Build history of the part. All positions in model axes, mm. Coordinates: 2 decimals unless noted, no trailing zeros. Order: outer loops, then holes, each group sorted by start corner. A loop starts at its lowest first (then second) coordinate and runs counter-clockwise, first axis right, second up. Notation, with made-up numbers: (51.5, 52) - (102.5, 52) arc R30 ccw to (102.5, 91) - close; hole circle Ø10 at (-33, -36). An arc over 180 degrees is marked (long way). Return JSON: item names as keys, results as strings.
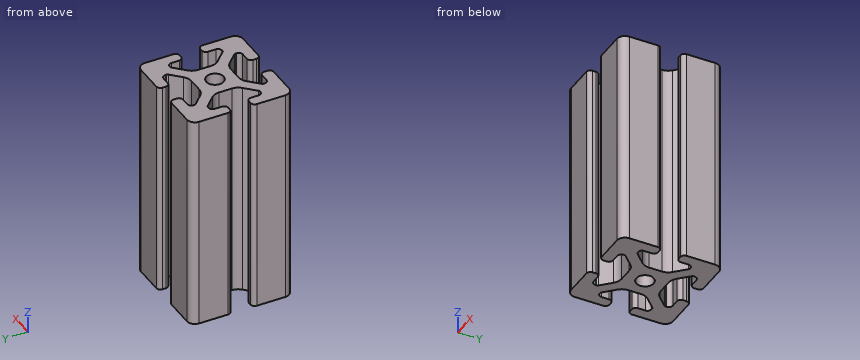
from build123d import *

# Parameters (mm, degrees)
SKETCH1_R      = 3.4
EXTRUDE1_DEPTH = 85.4


with BuildPart() as part:
    # Sketch1 → Extrude1 (new body)
    with BuildSketch(Plane.XY):
        with BuildLine():
            Line((-8.715, -15.524615034), (-5.63, -15.524615034))
            ThreePointArc((-5.63, -15.524615034), (-4.519842354, -15.984457388), (-4.06, -17.094615034))
            Line((-4.06, -17.094615034), (-4.06, -18.43))
            ThreePointArc((-4.06, -18.43), (-4.519842354, -19.540157646), (-5.63, -20))
            Line((-5.63, -20), (-16.674615034, -20))
            ThreePointArc((-16.674615034, -20), (-18.951578385, -19.194274381), (-20, -17.018368134))
            Line((-20, -17.018368134), (-20, -5.757918808))
            ThreePointArc((-20, -5.757918808), (-19.564709668, -4.603883664), (-18.43, -4.120449326))
            Line((-18.43, -4.120449326), (-17.25, -4.120449326))
            ThreePointArc((-17.25, -4.120449326), (-16.115287682, -4.60388249), (-15.67999625, -5.757919334))
            Line((-15.67999625, -5.757919334), (-15.67999625, -8.715399492))
            ThreePointArc((-15.67999625, -8.715399492), (-15.220153896, -9.825557139), (-14.10999625, -10.285399492))
            Line((-14.10999625, -10.285399492), (-13.816898819, -10.285399492))
            ThreePointArc((-13.816898819, -10.285399492), (-13.526061711, -10.227547119), (-13.279501941, -10.062800646))
            Line((-13.279501941, -10.062800646), (-9.076242789, -5.859541495))
            ThreePointArc((-9.076242789, -5.859541495), (-8.046572221, -4.318530588), (-7.685, -2.500784284))
            Line((-7.685, -2.500784284), (-7.685, 2.500784284))
            ThreePointArc((-7.685, 2.500784284), (-8.046572221, 4.318530588), (-9.076242789, 5.859541495))
            Line((-9.076242789, 5.859541495), (-13.040489136, 9.823787841))
            ThreePointArc((-13.040489136, 9.823787841), (-13.354224618, 10.012729352), (-13.71989919, 10.033001362))
            Line((-13.71989919, 10.033001362), (-14.05520779, 10.044710596))
            ThreePointArc((-14.05520779, 10.044710596), (-15.200613642, 9.605030484), (-15.68, 8.475666998))
            Line((-15.68, 8.475666998), (-15.68, 5.572979049))
            ThreePointArc((-15.68, 5.572979049), (-16.139842354, 4.462821403), (-17.25, 4.002979049))
            Line((-17.25, 4.002979049), (-18.43, 4.002979049))
            ThreePointArc((-18.43, 4.002979049), (-19.540157646, 4.462821403), (-20, 5.572979049))
            Line((-20, 5.572979049), (-20, 13.004526564))
            Line((-20, 13.004526564), (-20, 16.83))
            ThreePointArc((-20, 16.83), (-19.071528496, 19.071528496), (-16.83, 20))
            Line((-16.83, 20), (-5.63, 20))
            ThreePointArc((-5.63, 20), (-4.519842354, 19.540157646), (-4.06, 18.43))
            Line((-4.06, 18.43), (-4.06, 17.094615034))
            ThreePointArc((-4.06, 17.094615034), (-4.519842354, 15.984457388), (-5.63, 15.524615034))
            Line((-5.63, 15.524615034), (-8.715, 15.524615034))
            ThreePointArc((-8.715, 15.524615034), (-9.825157646, 15.06477268), (-10.285, 13.954615034))
            Line((-10.285, 13.954615034), (-10.285, 13.492503602))
            ThreePointArc((-10.285, 13.492503602), (-10.227148445, 13.201664194), (-10.062401154, 12.955102448))
            Line((-10.062401154, 12.955102448), (-6.217092793, 9.109794088))
            ThreePointArc((-6.217092793, 9.109794088), (-4.63891877, 8.055291919), (-2.777335583, 7.685))
            Line((-2.777335583, 7.685), (2.777335583, 7.685))
            ThreePointArc((2.777335583, 7.685), (4.63891877, 8.055291919), (6.217092793, 9.109794088))
            Line((6.217092793, 9.109794088), (10.062401154, 12.955102448))
            ThreePointArc((10.062401154, 12.955102448), (10.227148445, 13.201664194), (10.285, 13.492503602))
            Line((10.285, 13.492503602), (10.285, 13.954615034))
            ThreePointArc((10.285, 13.954615034), (9.825157646, 15.06477268), (8.715, 15.524615034))
            Line((8.715, 15.524615034), (5.63, 15.524615034))
            ThreePointArc((5.63, 15.524615034), (4.519842354, 15.984457388), (4.06, 17.094615034))
            Line((4.06, 17.094615034), (4.06, 18.43))
            ThreePointArc((4.06, 18.43), (4.519842354, 19.540157646), (5.63, 20))
            Line((5.63, 20), (12.979635074, 20))
            Line((12.979635074, 20), (16.83, 20))
            ThreePointArc((16.83, 20), (19.071528496, 19.071528496), (20, 16.83))
            Line((20, 16.83), (20, 13.001098436))
            Line((20, 13.001098436), (20, 5.63))
            ThreePointArc((20, 5.63), (19.540157461, 4.519842693), (18.43, 4.060000526))
            Line((18.43, 4.060000526), (17.24999625, 4.060000526))
            ThreePointArc((17.24999625, 4.060000526), (16.139838603, 4.519842879), (15.67999625, 5.630000526))
            Line((15.67999625, 5.630000526), (15.67999625, 8.715399492))
            ThreePointArc((15.67999625, 8.715399492), (15.220153896, 9.825557139), (14.10999625, 10.285399492))
            Line((14.10999625, 10.285399492), (13.816903094, 10.285399492))
            ThreePointArc((13.816903094, 10.285399492), (13.526063686, 10.227547937), (13.279501941, 10.062800646))
            Line((13.279501941, 10.062800646), (9.076242789, 5.859541495))
            ThreePointArc((9.076242789, 5.859541495), (8.046572221, 4.318530588), (7.685, 2.500784284))
            Line((7.685, 2.500784284), (7.685, -2.500784284))
            ThreePointArc((7.685, -2.500784284), (8.046572221, -4.318530588), (9.076242789, -5.859541495))
            Line((9.076242789, -5.859541495), (13.163657296, -9.946956002))
            ThreePointArc((13.163657296, -9.946956002), (13.35903797, -10.160433474), (13.6200547, -10.285399492))
            Line((13.6200547, -10.285399492), (14.10999625, -10.285399492))
            ThreePointArc((14.10999625, -10.285399492), (15.220153896, -9.825557139), (15.67999625, -8.715399492))
            Line((15.67999625, -8.715399492), (15.67999625, -5.630000526))
            ThreePointArc((15.67999625, -5.630000526), (16.139838603, -4.519842879), (17.24999625, -4.060000526))
            Line((17.24999625, -4.060000526), (18.43, -4.060000526))
            ThreePointArc((18.43, -4.060000526), (19.540157461, -4.519842693), (20, -5.63))
            Line((20, -5.63), (20, -16.83))
            ThreePointArc((20, -16.83), (19.071528496, -19.071528496), (16.83, -20))
            Line((16.83, -20), (13, -20))
            Line((13, -20), (5.63, -20))
            ThreePointArc((5.63, -20), (4.519842354, -19.540157646), (4.06, -18.43))
            Line((4.06, -18.43), (4.06, -17.094615034))
            ThreePointArc((4.06, -17.094615034), (4.519842354, -15.984457388), (5.63, -15.524615034))
            Line((5.63, -15.524615034), (8.715, -15.524615034))
            ThreePointArc((8.715, -15.524615034), (9.825157646, -15.06477268), (10.285, -13.954615034))
            Line((10.285, -13.954615034), (10.285, -13.492503602))
            ThreePointArc((10.285, -13.492503602), (10.227148445, -13.201664194), (10.062401154, -12.955102448))
            Line((10.062401154, -12.955102448), (6.217092793, -9.109794088))
            ThreePointArc((6.217092793, -9.109794088), (4.63891877, -8.055291919), (2.777335583, -7.685))
            Line((2.777335583, -7.685), (-2.777335583, -7.685))
            ThreePointArc((-2.777335583, -7.685), (-4.63891877, -8.055291919), (-6.217092793, -9.109794088))
            Line((-6.217092793, -9.109794088), (-10.062401154, -12.955102448))
            ThreePointArc((-10.062401154, -12.955102448), (-10.227148445, -13.201664194), (-10.285, -13.492503602))
            Line((-10.285, -13.492503602), (-10.285, -13.954615034))
            ThreePointArc((-10.285, -13.954615034), (-9.825157646, -15.06477268), (-8.715, -15.524615034))
        make_face()
        Circle(SKETCH1_R, mode=Mode.SUBTRACT)
    extrude(amount=-EXTRUDE1_DEPTH)


solid = part.part
1. Drop flat-ended pins along their axis: pin 1 (0.7 mm diameter, centred on y = -18, z = -38, fed in from +X); pin 2 (5.5 mm diameter, centred on x = -12, z = -52, fed in from -Y); pin 3 (0.9 mm diameter, centred on x = -18, z = -25.5, fed in from -Y); pin 4 (8 mm diameter, centred on x = -9, y = -9, fed in from +Z). Give the stop position or say it passes through.
Check values:
{"pin 1": "x = 19.89", "pin 2": "y = -20", "pin 3": "y = -19.92", "pin 4": "z = 0"}
2. Probe L1, parallel to X at y = 17, z = -46; L2, parallel to Y at x = 14, z = -10.5; L3, parallel to X at y = 9, z = -52.5. List the from-to ranges inside material, lowest first.
Check values:
{"L1": "-20 to -4.06, 4.06 to 20", "L2": "-20 to -10.29, 10.29 to 20", "L3": "-20 to -15.59, -12.22 to -6.1, 6.1 to 12.22, 15.65 to 20"}
3. Cut at A-A on x = 0. Give the cut face in (y, z) (3 decimals), plus the area to 3 significant figures.
Check values:
{"outline": "(-7.685, -85.4) - (-3.4, -85.4) - (-3.4, 0) - (-7.685, 0) - close; (3.4, -85.4) - (7.685, -85.4) - (7.685, 0) - (3.4, 0) - close", "area": "732 mm²"}
